```python
from build123d import *

# Parameters (mm, degrees)
SKETCH1_R           = 7.5
BOSS_EXTRUDE1_DEPTH = 1.25


with BuildPart() as part:
    # Sketch1 → Boss-Extrude1 (new body, symmetric)
    with BuildSketch(Plane.XY):
        Polygon((0, 10.969655115), (-9.5, 5.484827557), (-9.5, -5.484827557), (0, -10.969655115), (9.5, -5.484827557), (9.5, 5.484827557), align=None)
        Circle(SKETCH1_R, mode=Mode.SUBTRACT)
    extrude(amount=BOSS_EXTRUDE1_DEPTH, both=True)

    # Sketch2 → Cut-Revolve1 (revolve, cut)
    with BuildSketch(Plane(origin=(0, 0, 0), x_dir=(1, 0, 0), z_dir=(0, 1, 0))):
        Polygon((-9.5, 1.25), (-12.977549271, -0.757764008), (-12.977549271, 1.25), align=None)
    revolve(axis=Axis((0, 0, 0), (0, 0, -1)), mode=Mode.SUBTRACT)


solid = part.part
```
Geometry check sheet. Reference: the model listing, model coordinates, mm. Coordinates: 2 decimals unless noted, no trailing zeros. Order: outer loops, then holes, each group sorted by start corner. A loop starts at its lowest first (then second) coordinate and runs counter-clockwise, first axis right, second up. Notation, with made-up numbers: (20.25, 40) - (74.25, 40) arc R32 ccw to (74.25, 70) - close; hole circle Ø10 at (56.5, -36.75). An arc over 180 degrees is marked (long way). Answer in a Markdown table with one row per item. Add a question column.
1. Material ranges on L1, parallel to X at y = -0.25, z = -0.3; L2, parallel to X at y = -3.25, z = -0.9; L3, parallel to Y at x = 0, z = -0.7, recorded low to high. Write a range as [from, to].
2. Gauge pin test, flat ends, axial feed: pin 1 Ø1.5 at (x, z) = (5.5, 0.5) entering from -Y; pin 2 Ø9 at (x, y) = (0, 0) entering from +Z. Record the tip position at first contact, or that the pin passes through.
3. Section check A-A (z = -0.05). Enter the section's corners in (x, y).
4. Draft check along X on faces 1 (the face through (-7.493, 0.33, -0.018)), 2 (the face through (4.684, -8.266, 0.018)), 3 (the face through (-4.8, -8.2, 0)), 4 (the face through (1, 8, -1.25)). Enter one of: +X half, -X half, draft (parallel to the pull), parting line (faces both ways), or undercut.
Data:
| question | item | result |
|---|---|---|
| 1 | L1 | x = [-9.5, -7.5], [7.5, 9.5] |
| 1 | L2 | x = [-9.5, -6.76], [6.76, 9.5] |
| 1 | L3 | y = [-10.45, -7.5], [7.5, 10.45] |
| 2 | pin 1 | stops at y = -8.23 |
| 2 | pin 2 | passes through |
| 3 | outline | (-9.5, -5.48) - (0, -10.97) - (9.5, -5.48) - (9.5, 5.48) - (0, 10.97) - (-9.5, 5.48) - close; hole circle Ø15 at (0, 0) |
| 4 | face 1 | undercut |
| 4 | face 2 | +X half |
| 4 | face 3 | -X half |
| 4 | face 4 | draft |
